```python
from build123d import *

# Parameters (mm, degrees)
SKETCH1_R               = 571.5
SKETCH1_R_2             = 469.9
BOSS_EXTRUDE1_DEPTH     = 114.3
BOSS_EXTRUDE2_START     = -107.95
BOSS_EXTRUDE2_DEPTH     = 107.95
CIRPATTERN2_COUNT       = 8
SKETCH18_R              = 457.217714823
SKETCH17_R              = 127
SKETCH9_R               = 127
BOSS_EXTRUDE4_DEPTH     = 76.2
SKETCH10_R              = 127
BOSS_EXTRUDE6_DEPTH     = 127
BOSS_EXTRUDE6_TAPER     = 9.74
FILLET1_R               = 19.05
SKETCH13_R              = 44.45
CUT_EXTRUDE2_DEPTH      = 50.8
BOSS_EXTRUDE9_START     = 71.12
BOSS_EXTRUDE9_DEPTH     = 71.12
CUT_EXTRUDE3_DEPTH      = 71.12
CUT_EXTRUDE3_DEPTH_BACK = 71.12
SKETCH19_R              = 63.5
CUT_EXTRUDE4_DEPTH      = 25.4


with BuildPart() as part:
    # Sketch1 → Boss-Extrude1 (new body)
    with BuildSketch(Plane.XY):
        Circle(SKETCH1_R)
        Circle(SKETCH1_R_2, mode=Mode.SUBTRACT)
    extrude(amount=BOSS_EXTRUDE1_DEPTH)

    # Sketch2 → Boss-Extrude2 (add)
    with BuildSketch(Plane.XY.offset(114.3).offset(BOSS_EXTRUDE2_START)):
        with BuildLine():
            ThreePointArc((76.2, 463.680461094), (0, 469.9), (-76.2, 463.680461094))
            Line((-76.2, 463.680461094), (-38.1, 121.15027858))
            ThreePointArc((-38.1, 121.15027858), (0, 127), (38.1, 121.15027858))
            Line((38.1, 121.15027858), (76.2, 463.680461094))
        make_face()
    boss_extrude2 = extrude(amount=BOSS_EXTRUDE2_DEPTH)

    # CirPattern2: Boss-Extrude2 ×8 about axis
    cirpattern2_axis = Axis((0, 0, 0), (0, 0, 1))
    for i in range(1, CIRPATTERN2_COUNT):
        add(boss_extrude2.rotate(cirpattern2_axis, i * 360 / CIRPATTERN2_COUNT))

    # Sketch18 → Cut-Loft1 section 0
    with BuildSketch(Plane.XY.offset(114.3)):
        Circle(SKETCH18_R)
    # Sketch17 → Cut-Loft1 section 1
    with BuildSketch(Plane.XY.offset(76.2)):
        Circle(SKETCH17_R)
    loft(mode=Mode.SUBTRACT)

    # Sketch9 → Boss-Extrude4 (add)
    with BuildSketch(Plane.XY):
        with Locations(Location((0, 0, 0), (0, 0, 162.542396876))):
            Circle(SKETCH9_R)
    extrude(amount=BOSS_EXTRUDE4_DEPTH)

    # Sketch10 → Boss-Extrude6 (add)
    with BuildSketch(Plane.XY.offset(76.2)):
        with Locations(Location((0, 0, 0), (0, 0, 162.542396876))):
            Circle(SKETCH10_R)
    extrude(amount=BOSS_EXTRUDE6_DEPTH, taper=BOSS_EXTRUDE6_TAPER)

    # Fillet1
    fillet1_edges = [part.edges().sort_by_distance(p)[0] for p in [
        (100.35462173, -31.560068477, 203.2),
    ]]
    fillet(fillet1_edges, radius=FILLET1_R)

    # Sketch13 → Cut-Extrude2 (cut)
    with BuildSketch(Plane.XY.offset(203.2)):
        Circle(SKETCH13_R)
    extrude(amount=-CUT_EXTRUDE2_DEPTH, mode=Mode.SUBTRACT)

    # Sketch15 → Boss-Extrude9 (add)
    with BuildSketch(Plane.XY.offset(152.4).offset(BOSS_EXTRUDE9_START)):
        with BuildLine():
            Line((-9.525, 43.417472001), (-9.525, 30.287569645))
            ThreePointArc((-9.525, 30.287569645), (-31.75, 0), (-9.525, -30.287569645))
            Line((-9.525, -30.287569645), (-9.525, -43.417472001))
            ThreePointArc((-9.525, -43.417472001), (0, -44.45), (9.525, -43.417472001))
            Line((9.525, -43.417472001), (9.525, -30.287569645))
            ThreePointArc((9.525, -30.287569645), (31.75, 0), (9.525, 30.287569645))
            Line((9.525, 30.287569645), (9.525, 43.417472001))
            ThreePointArc((9.525, 43.417472001), (0, 44.45), (-9.525, 43.417472001))
        make_face()
    extrude(amount=-BOSS_EXTRUDE9_DEPTH)

    # Sketch16 → Cut-Extrude3 (cut, two sides: drawn at the far end of the back side and taken through both)
    with BuildSketch(Plane(origin=(0, 0, 0), x_dir=(0, 0, -1), z_dir=(1, 0, 0)).offset(-CUT_EXTRUDE3_DEPTH_BACK)):
        Polygon((-223.52, 30.287569645), (-208.28, 44.45), (-223.52, 44.45), align=None)
        Polygon((-223.52, -44.45), (-223.52, -30.287569645), (-208.28, -44.45), align=None)
    extrude(amount=CUT_EXTRUDE3_DEPTH + CUT_EXTRUDE3_DEPTH_BACK, mode=Mode.SUBTRACT)

    # Sketch19 → Cut-Extrude4 (cut)
    with BuildSketch(Plane(origin=(0, 0, 0), x_dir=(-1, 0, 0), z_dir=(0, 0, -1))):
        Circle(SKETCH19_R)
    extrude(amount=-CUT_EXTRUDE4_DEPTH, mode=Mode.SUBTRACT)


solid = part.part
```
For this review, take the finished solid that the model builds, in its own axes (mm). A direction names the side the tool comes from. Give positions to 0.01 mm unless a question says otherwise; leave off trailing zeros. Write each loop counter-clockwise with the first axis right and the second up, starting at its lowest first coordinate (ties: lowest second). Pieces come first, ordered by that corner, then holes. Notation, with made-up numbers: M -23,25.25 L -10,25.25 A20 cw -10,49.25 Z; hole C -37,19 d7. An arc over 180 degrees is marked long. One line per item, written item: value.
1) For P1, Ø12, axis at y = 107.5, z = 138, coming from the +X side; P2, Ø4, axis at y = -36.5, z = 203, coming from the -X side; P3, Ø10, axis at x = 49, y = 4, coming from the +Z side, all flat-tipped, find the tip position at first contact; note any pin that passes through.
Results are:
P1: stops at x = 57.17
P2: stops at x = -91.06
P3: stops at z = 203.2
2) The part is to be moulded in two halves that separate along X. For faces 5 (the cylindrical face through (-570.947, 25.128, 56.35)), 6 (the cylindrical face through (-44.442, 0.843, 178.156)), 7 (the flat face through (-30, -33.4, 203.2)), say which applies: +X half, -X half, draft (parallel to the pull), parting line (faces both ways), or undercut.
Results are:
face 5: parting line
face 6: undercut
face 7: draft
3) For faces 1 (the conical face through (1.08, 253.1, 90.75)), 2 (the flat face through (245.296, 164.851, 47.575)), 3 (the flat face through (239, -237, 6.35)), 4 (the flat face through (0, 0, 223.52)), list the 3-axis set-ups (+Z, -Z, +X, -X, +Y, -Y) from which the entire face can be reached by the end or side of a thin tool; tool diameter is ignored.
Results are:
face 1: +Z
face 2: +Z, -Z
face 3: -Z
face 4: +Z, +X, -X, +Y, -Y
4) Take a section at B-B, the plane y = 180.5. Count the separate pieces of the cut face and the enclosed holes in it, then the cut area to 3 significant figures.
Results are:
separate pieces: 5
enclosed holes: 0
area: 57,600 mm²
5) For line 1 (Y direction, x = 0, z = 6); line 2 (X direction, y = 270, z = 18.5); line 3 (Y direction, x = 0, z = 11), list the stretches that pass through material, from the lowest coordinate up. Write a range as from..to.
Results are:
line 1: y = -571.5..-469.9, -127..-63.5, 63.5..127, 469.9..571.5
line 2: x = -503.7..-384.59, -376.76..-184.61, -54.66..54.66, 184.61..376.76, 384.59..503.7
line 3: y = -571.5..-63.5, 63.5..571.5
6) Take a section at D-D, the plane y = -491. Write out the cut boundary in (x, z).
Results are:
outline: M -292.46,0 L 292.46,0 L 292.46,114.3 L -292.46,114.3 Z
